Build history of the part. All positions in model axes, mm. A direction names the side the tool comes from. Give positions to 0.01 mm unless a question says otherwise; leave off trailing zeros. Order: outer loops, then holes, each group sorted by start corner. A loop starts at its lowest first (then second) coordinate and runs counter-clockwise, first axis right, second up. Notation, with made-up numbers: (-33.75, -36.5) - (-11.75, -36.5) arc R17 ccw to (-11.75, -32.5) - close; hole circle Ø4 at (73.5, 60). An arc over 180 degrees is marked (long way). One line per item, written item: value.
```python
from build123d import *

# Parameters (mm, degrees)
SKETCH1_R           = 7.5
BOSS_EXTRUDE1_DEPTH = 5
SKETCH6_R           = 1
SKETCH12_R          = 4.15
BOSS_EXTRUDE2_DEPTH = 3
SKETCH13_R          = 1.5
BOSS_EXTRUDE3_DEPTH = 14.5
CUT_EXTRUDE5_REACH  = 24.5
SKETCH21_R          = 1
SKETCH22_R          = 0.75
CUT_EXTRUDE6_DEPTH  = 18.5000001
SKETCH23_R          = 0.654937639
SKETCH23_R_2        = 0.75
CUT_EXTRUDE7_DEPTH  = 10


with BuildPart() as part:
    # Sketch1 → Boss-Extrude1 (new body)
    with BuildSketch(Plane(origin=(0, 0, 0), x_dir=(1, 0, 0), z_dir=(0, 1, 0))):
        Circle(SKETCH1_R)
    extrude(amount=BOSS_EXTRUDE1_DEPTH)

    # Cut-Sweep2: sweep along a path in Sketch5
    with BuildLine(Plane.XY) as cut_sweep2_path:
        Line((0, 0), (0, 0.5))
        ThreePointArc((0, 0.5), (0.878679656, 2.621320344), (3, 3.5))
        Line((3, 3.5), (7.5, 3.5))
    # Sketch6 → Cut-Sweep2 (sweep, cut)
    with BuildSketch(Plane(origin=(0, 0, 0), x_dir=(-1, 0, 0), z_dir=(0, -1, 0))):
        Circle(SKETCH6_R)
    sweep(path=cut_sweep2_path.line, mode=Mode.SUBTRACT)

    # Sketch12 → Boss-Extrude2 (add)
    with BuildSketch(Plane(origin=(0, 0, 0), x_dir=(-1, 0, 0), z_dir=(0, -1, 0))):
        Circle(SKETCH12_R)
    extrude(amount=BOSS_EXTRUDE2_DEPTH)

    # Sketch13 → Boss-Extrude3 (add)
    with BuildSketch(Plane.XZ.offset(3)):
        Circle(SKETCH13_R)
    extrude(amount=BOSS_EXTRUDE3_DEPTH)

    # Sketch21 → Cut-Extrude5 (cut, up to next)
    with BuildSketch(Plane(origin=(0, -17.5, 0), x_dir=(-1, 0, 0), z_dir=(0, -1, 0)), mode=Mode.PRIVATE) as cut_extrude5_sk1:
        Circle(SKETCH21_R)
    cut_extrude5_tool1 = extrude(cut_extrude5_sk1.sketch, amount=-CUT_EXTRUDE5_REACH, mode=Mode.PRIVATE) & part.part
    add(cut_extrude5_tool1.solids().sort_by_distance((0, -17.5, 0))[0], mode=Mode.SUBTRACT)

    # Sketch22 → Cut-Extrude6 (cut, through all)
    with BuildSketch(Plane(origin=(10, 0, 0), x_dir=(0, 0, -1), z_dir=(1, 0, 0))):
        with Locations((0, -16)):
            Circle(SKETCH22_R)
    extrude(amount=-CUT_EXTRUDE6_DEPTH, mode=Mode.SUBTRACT)

    # Sketch23 → Cut-Extrude7 (cut)
    with BuildSketch(Plane.XZ.offset(3)):
        with Locations((0, 3)):
            Circle(SKETCH23_R)
        with Locations((0, -3)):
            Circle(SKETCH23_R_2)
    extrude(amount=-CUT_EXTRUDE7_DEPTH, mode=Mode.SUBTRACT)


solid = part.part
```
(1) Drill centre lines: line 1 (Z direction, x = 0, y = -10.25); line 2 (Z direction, x = 0, y = -2.75); line 3 (Z direction, x = 0, y = 0.25). Where is each one in solid material? Low to high.
Completed:
line 1: -1.5 to -1, 1 to 1.5
line 2: -4.15 to -3.75, -2.25 to -1, 1 to 2.35, 3.65 to 4.15
line 3: -7.5 to -3.75, -2.25 to -1, 1 to 2.35, 3.65 to 7.5
(2) Slice it at B-B, the plane y = -7.5. Give the cut face in (x, z).
Completed:
outline: circle Ø3 at (0, 0); hole circle Ø2 at (0, 0)
(3) Slice it at D-D, the plane y = -1.5. Give the cut face in (x, z).
Completed:
outline: circle Ø8.3 at (0, 0); hole circle Ø2 at (0, 0); hole circle Ø1.5 at (0, -3); hole circle Ø1.31 at (0, 3)
(4) Slice it at A-A, the plane z = 0. Give the cut face in (x, y).
Completed:
outline: (-7.5, 0) - (-4.15, 0) - (-4.15, -3) - (-1.5, -3) - (-1.5, -15.25) - (-1, -15.25) - (-1, 0.5) arc R4 cw to (3, 4.5) - (7.5, 4.5) - (7.5, 5) - (-7.5, 5) - close; (-1.5, -17.5) - (-1, -17.5) - (-1, -16.75) - (-1.5, -16.75) - close; (1, -17.5) - (1.5, -17.5) - (1.5, -16.75) - (1, -16.75) - close; (1, -15.25) - (1.5, -15.25) - (1.5, -3) - (4.15, -3) - (4.15, 0) - (7.5, 0) - (7.5, 2.5) - (3, 2.5) arc R2 ccw to (1, 0.5) - close
(5) Pull direction Y, two halves, no side cores. Call faces 4 (the face through (-0.163, 0.944, -3.732)), 5 (the face through (3.2, 0, 3.2)), 6 (the face through (0, 5, 0)), 7 (the face through (1.087, -16.456, 0.595)): +Y half, -Y half, draft (parallel to the pull), parting line (faces both ways), or undercut.
Completed:
face 4: draft
face 5: -Y half
face 6: +Y half
face 7: undercut
(6) 3-axis set-ups, long thin cutter, end or side, ignore diameter. For faces 1 (the face through (-7.493, 2.465, -0.33)), 2 (the face through (0.9, -1.48, 4.05)), 3 (the face through (5.3, 2.5, 0)): which of +Z, -Z, +X, -X, +Y, -Y reach the whole face in a straight line?
Completed:
face 1: +Y, -Y
face 2: -Y
face 3: +X
(7) Slice it at C-C, the plane x = 0. Count the separate pieces of the cut face and the enclosed holes in it, and give its area (3 significant figures).
Completed:
separate pieces: 3
enclosed holes: 0
area: 80.4 mm²
(8) Pin check, flat tips, straight feed: P1, Ø1.4, axis at y = -16, z = 0, coming from the +X side; P2, Ø2, axis at y = -2, z = -1.5, coming from the -X side; P3, Ø2, axis at y = -16, z = 0, coming from the +X side; P4, Ø4, axis at x = 0, z = 5.5, coming from the -Y side. Stop position of each tip, or through.
Completed:
P1: through
P2: x = -4.12
P3: x = 1.5
P4: y = -3
